Design review of the part built by this model. Coordinates are the model's own, in mm. A direction names the side the tool comes from. Coordinates: 2 decimals unless noted, no trailing zeros. Loops run counter-clockwise (first coordinate to the right, second up) from the corner with the lowest first, then second, coordinate; pieces in that order, holes last. Notation, with made-up numbers: (66, 1.5) -> (103, 1.5) arc R8 cw to (103, 9.5) -> close; hole circle Ø3 at (-34.5, 81.5). An arc over 180 degrees is marked (long way). One line per item, written item: value. Start each with the question number.
1. Insertion check: pin 1 (9.5 mm diameter, centred on y = 15.5, z = 25, fed in from +X); pin 2 (1.7 mm diameter, centred on x = 8, z = 38.5, fed in from -Y); pin 3 (5 mm diameter, centred on x = 28.5, y = -0.92, fed in from +Z); pin 4 (8 mm diameter, centred on x = 0, z = 5.5, fed in from +Y). Each pin has a flat end and moves straight along its axis. Give the tip position at first contact, or say it passes through.
2. Add section D-D on y = 8.25. Write out the cut boundary in (x, z), plus the area to 3 significant figures.
3. For probe 1 along X at (y, z) = (-1, 34.5); probe 2 along Y at (x, z) = (-3.5, 31.5); probe 3 along X at (y, z) = (-2.5, 35), list the stretches that pass through material, from the lowest coordinate up.
4. Draft analysis for pull direction X (two halves, no side actions). For faces 6 (the flat face through (12.3, 2.913, 38.4)), 7 (the flat face through (12, 1, 0)), state which applies: pulls with the +X half, pulls with the -X half, needs draft (parallel to the pull), parting line crosses it, or undercut.
5. Machinability: for faces 1 (the flat face through (12, 1, 39)), 2 (the flat face through (25, 2, 19)), 3 (the cylindrical face through (25.753, -1.043, 19.227)), 4 (the flat face through (12, 0, 38)), 5 (the cylindrical face through (25.989, 2.948, 19.227)), which of the approach directions +Z, -Z, +X, -X, +Y, -Y give a long, thin tool a straight path to every point of the face, cutting with its end or side? Answer none if there is none.
6. Add section C-C on y = -1.75. Write out the cut boundary in (x, z), plus the area to 3 significant figures.
7. Add section A-A on x = -3.5. Write out the cut boundary in (y, z), plus the area to 3 significant figures.
8. Add section B-B on z = 33.5. Write out the cut boundary in (x, y).
```python
from build123d import *

# Parameters (mm, degrees)
F1_DEPTH = 25
F2_R     = 2.75
F3_DEPTH = 39
F6_DEPTH = 39
F7_DEPTH = 25
F8_DEPTH = 1.4888694367


with BuildPart() as f1:
    # F0 (on Right) → F1 (new body)
    with BuildSketch(Plane.YZ):
        Polygon((18.5510310847, 29.8126723238), (0.5779567464, 0), (2.9132927302, 0), (21.5006141558, 30.8315490499), (0, 39), (0, 36.8605262312), align=None)
    extrude(amount=F1_DEPTH)

    # F2 (on face) → F3 (join)
    with BuildSketch(Plane(origin=(0, 0, 0), x_dir=(1, 0, 0), z_dir=(0, 0, -1))):
        with BuildLine():
            ThreePointArc((0.4764934301, -0.5779567464), (0.6810642831, 0.1596775533), (0.75, 0.9220432536))
            ThreePointArc((0.75, 0.9220432536), (-7.5581707702, 2.1844813709), (0, -1.4888694367))
            Line((0, -1.4888694367), (0, -0.5779567464))
            Line((0, -0.5779567464), (0.4764934301, -0.5779567464))
        make_face()
        with Locations((-3.5, 0.9220432536)):
            Circle(F2_R, mode=Mode.SUBTRACT)
        with BuildLine():
            Line((0, -0.5779567464), (0, -1.4888694367))
            ThreePointArc((0, -1.4888694367), (0.2658901982, -1.0478732459), (0.4764934301, -0.5779567464))
            Line((0.4764934301, -0.5779567464), (0, -0.5779567464))
        make_face()
        with BuildLine():
            ThreePointArc((32.75, 0.9220432536), (27.7376342997, 5.1031075366), (24.5235065699, -0.5779567464))
            Line((24.5235065699, -0.5779567464), (25, -0.5779567464))
            Line((25, -0.5779567464), (25, -1.4888694367))
            ThreePointArc((25, -1.4888694367), (29.7624381173, -3.1361275166), (32.75, 0.9220432536))
        make_face()
        with Locations((28.5, 0.9220432536)):
            Circle(F2_R, mode=Mode.SUBTRACT)
        with BuildLine():
            Line((25, -0.5779567464), (24.5235065699, -0.5779567464))
            ThreePointArc((24.5235065699, -0.5779567464), (24.7341098018, -1.0478732459), (25, -1.4888694367))
            Line((25, -1.4888694367), (25, -0.5779567464))
        make_face()
    extrude(amount=-F3_DEPTH)

    # F5 (on face) → F6 (join, through all)
    with BuildSketch(Plane(origin=(0, 0, 0), x_dir=(1, 0, 0), z_dir=(0, 0, -1))):
        with BuildLine():
            ThreePointArc((-2.0012357145, -3.0549160895), (-1.0031203269, -2.9487427884), (0, -2.9132927302))
            Line((0, -2.9132927302), (0, -1.4888694367))
            ThreePointArc((0, -1.4888694367), (-0.8808328375, -2.4249648693), (-2.0012357145, -3.0549160895))
        make_face()
        with BuildLine():
            Line((25, -1.4888694367), (25, -2.9132927302))
            ThreePointArc((25, -2.9132927302), (26.0031203269, -2.9487427884), (27.0012357145, -3.0549160895))
            ThreePointArc((27.0012357145, -3.0549160895), (25.8808328375, -2.4249648693), (25, -1.4888694367))
        make_face()
    extrude(amount=-F6_DEPTH)

    # F7 (add): a face of the model
    f7_faces = [f1.faces().sort_by_distance(p)[0] for p in [
        (0, 2.2778987033, 38.5672936668),
    ]]
    extrude(f7_faces, amount=F7_DEPTH)

    # F8 (add, through all): a face of the model
    f8_faces = [f1.faces().sort_by_distance(p)[0] for p in [
        (12.5, 1.4888694367, 38.7171765216),
    ]]
    extrude(f8_faces, amount=F8_DEPTH)


solid = f1.part
```
Worked answers:
1. pin 1: stops at x = 25
1. pin 2: stops at y = 0
1. pin 3: passes through
1. pin 4: stops at y = 8.64
2. outline: (0, 8.85) -> (25, 8.85) -> (25, 12.73) -> (0, 12.73) -> close; (0, 33.73) -> (25, 33.73) -> (25, 35.87) -> (0, 35.87) -> close
2. area: 150 mm²
3. probe 1: x = -7.75 to -6.25, -0.75 to 0.75, 24.25 to 25.75, 31.25 to 32.75
3. probe 2: y = -5.17 to -3.67, 1.83 to 3.33
3. probe 3: x = -7.45 to -5.75, -1.25 to 0.45, 24.55 to 26.25, 30.75 to 32.45
4. face 6: undercut
4. face 7: needs draft
5. face 1: +Z, +X, -X, +Y, -Y
5. face 2: none
5. face 3: +Z, -Z
5. face 4: +Z, -Z, -Y
5. face 5: +Z, -Z, +Y
6. outline: (-7.67, 0) -> (-6.12, 0) -> (-6.12, 39) -> (-7.67, 39) -> close; (-0.88, 0) -> (0.67, 0) -> (0.67, 39) -> (-0.88, 39) -> close; (24.33, 0) -> (25.88, 0) -> (25.88, 39) -> (24.33, 39) -> close; (31.12, 0) -> (32.67, 0) -> (32.67, 39) -> (31.12, 39) -> close
6. area: 241 mm²
7. outline: (-5.17, 0) -> (-3.67, 0) -> (-3.67, 39) -> (-5.17, 39) -> close; (1.83, 0) -> (3.33, 0) -> (3.33, 39) -> (1.83, 39) -> close
7. area: 117 mm²
8. outline: (-2, 3.05) arc R4.25 ccw (long way) to (0, 1.49) -> (0, 2.91) arc R14.21 cw to start; (0, 8.85) -> (25, 8.85) -> (25, 14.48) -> (0, 14.48) -> close; (25, 1.49) arc R4.25 ccw (long way) to (27, 3.05) arc R14.21 cw to (25, 2.91) -> close; hole circle Ø5.5 at (-3.5, -0.92); hole circle Ø5.5 at (28.5, -0.92)
